from build123d import *

# Parameters (mm, degrees)
FILLET1_R = 20
SHELL1_T  = -2.5


with BuildPart() as part:
    # Sketch2 → Revolve1 (revolve)
    with BuildSketch(Plane(origin=(0, 0, 0), x_dir=(1, 0, 0), z_dir=(0, 1, 0))):
        with BuildLine():
            Line((0, -108.5), (0, -6))
            Line((0, -6), (47.816178594, -6))
            Line((47.816178594, -6), (50, 0))
            Line((50, 0), (64, 0))
            Line((64, 0), (64, -15.8))
            Line((64, -15.8), (46.137243112, -94.742026455))
            ThreePointArc((46.137243112, -94.742026455), (44.738953709, -98.818081472), (42.5, -102.5))
            Line((42.5, -102.5), (42.5, -108.5))
            Line((42.5, -108.5), (0, -108.5))
        make_face()
    revolve(axis=Axis((0, 0, 108.5), (0, 0, -1)))

    # Fillet1
    fillet1_edges = [part.edges().sort_by_distance(p)[0] for p in [
        (-64, 0, 15.8),
    ]]
    fillet(fillet1_edges, radius=FILLET1_R)

    # Shell1
    shell1_openings = [part.faces().sort_by_distance(p)[0] for p in [
        (0, 0, 108.5),
    ]]
    offset(amount=SHELL1_T, openings=shell1_openings, kind=Kind.INTERSECTION)


solid = part.part
Input: part model. Units: mm. Frame: model coordinates. A direction names the side the tool comes from. Coordinates: 2 decimals unless noted, no trailing zeros. Loops run counter-clockwise (first coordinate to the right, second up) from the corner with the lowest first, then second, coordinate; pieces in that order, holes last.
(1) Section A-A on z = 35. Return the cut outline in (x, y), then the cut area to 3 significant figures.
(2) Section B-B on z = 49. Return the cut outline in (x, y).
(3) Pull-direction query (Y, two-part tool) for faces 1 (the face through (58.66, -18.47, 8.11)), 2 (the face through (-29, 28, 108.5)), 3 (the face through (59.12, 24.51, 6.88)); classes: released by +Y, released by -Y, zero draft, split by the parting line, or undercut.
(4) First-contact query: pin 1 Ø6 at (y, z) = (-44, 59.5) entering from -X; pin 2 Ø1.5 at (y, z) = (-18, 32) entering from +X; pin 3 Ø1 at (x, y) = (0, 4.5) entering from +Z. Flat tips, straight axial feed; report the tip coordinate or a pass-through.
(5) Material intervals for probe 1 along Y at (x, z) = (0, 106); probe 2 along Y at (x, z) = (0, 8); probe 3 along X at (y, z) = (0, 6.75), sorted ascending.
(6) Set-up query: faces 4 (the face through (1, -1, 6)), 5 (the face through (-33.727, 25.861, 105.542)), 6 (the face through (47.41, -14.93, 8.12)). Return all of +Z, -Z, +X, -X, +Y, -Y with unobstructed straight access to the full face (end or side cutting, diameter ignored); none if empty.
Data:
1. outline: circle Ø119.31 at (0, 0); hole circle Ø114.18 at (0, 0)
1. area: 940 mm2
2. outline: circle Ø112.98 at (0, 0); hole circle Ø107.85 at (0, 0)
3. face 1: undercut
3. face 2: zero draft
3. face 3: split by the parting line
4. pin 1: stops at x = -35.47
4. pin 2: stops at x = 57.88
4. pin 3: stops at z = 8.5
5. probe 1: y = -42.5 to -40, 40 to 42.5
5. probe 2: y = -64 to -61.5, -49.75 to 49.75, 61.5 to 64
5. probe 3: x = -64 to -61.5, -50.2 to 50.2, 61.5 to 64
6. face 4: -Z
6. face 5: +Z
6. face 6: none
